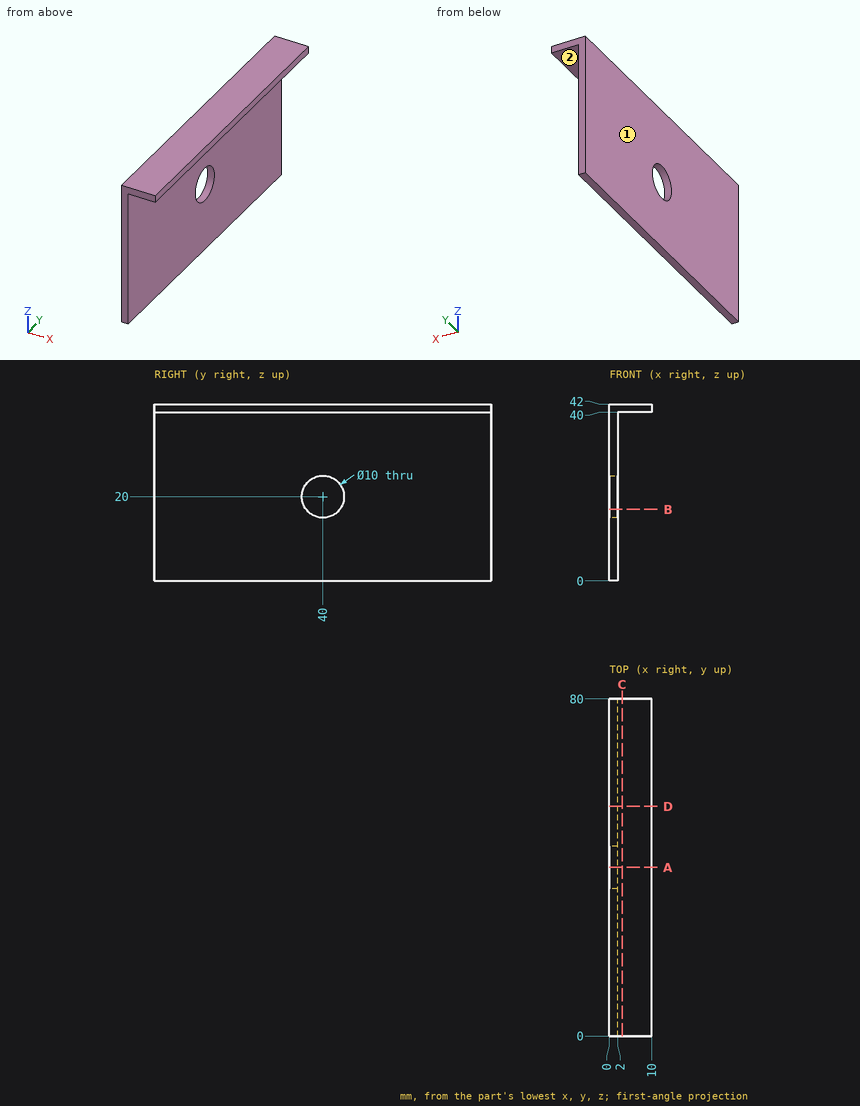
Job drawing, mm, ordinate dimensions from the low corner. One solid piece. A direction names the side the tool comes from. Give positions to 0.01 mm unless a question says otherwise; leave off trailing zeros. Loops run counter-clockwise (first coordinate to the right, second up) from the corner with the lowest first, then second, coordinate; pieces in that order, holes last. Notation, with made-up numbers: M -8.75,-31.5 L 10.25,-31.5 A18 ccw 10.25,-9.5 Z; hole C -37.5,5.25 d10. An arc over 180 degrees is marked long. Answer in a Markdown table with one row per item. Add a question column.
Item 1: Band-saw the part on A-A on y = 40. Give the cut face in (x, z).
Item 2: Drop a flat-ended pin along its axis: P1, Ø2.5, axis at x = 4, y = 21.5, coming from the -Z side. Give the stop position or say it passes through.
Item 3: Band-saw the part on C-C on x = 3. Give the cut face in (y, z).
Item 4: Probe probe 1 along Y at (x, z) = (1, 20); probe 2 along Z at (x, y) = (6.75, 28.5); probe 3 along X at (y, z) = (27.5, 28). List the from-to ranges inside material, lowest first.
Item 5: Band-saw the part on D-D on y = 54.5. Give the cut face in (x, z), then the cut area to 3 significant figures.
Item 6: Band-saw the part on B-B on z = 17. Give the cut face in (x, y).
Item 7: Tool access for the marked faces 1 and 2: list every direction of +Z, -Z, +X, -X, +Y, -Y with a clear straight run to the whole face (end or side of a thin tool).
Reply:
| question | item | result |
|---|---|---|
| 1 | outline | M 0,0 L 2,0 L 2,15 L 0,15 Z; M 0,25 L 2,25 L 2,40 L 10,40 L 10,42 L 0,42 Z |
| 2 | P1 | stops at z = 40 |
| 3 | outline | M 0,40 L 80,40 L 80,42 L 0,42 Z |
| 4 | probe 1 | y = 0 to 35, 45 to 80 |
| 4 | probe 2 | z = 40 to 42 |
| 4 | probe 3 | x = 0 to 2 |
| 5 | outline | M 0,0 L 2,0 L 2,40 L 10,40 L 10,42 L 0,42 Z |
| 5 | area | 100 mm^2 |
| 6 | outline | M 0,0 L 2,0 L 2,36 L 0,36 Z; M 0,44 L 2,44 L 2,80 L 0,80 Z |
| 7 | face 1 | +Z, -Z, -X, +Y, -Y |
| 7 | face 2 | -Z, +X, +Y, -Y |
